Work out the finished part from the listing and answer in its coordinate system (mm). A direction names the side the tool comes from. Coordinates: 2 decimals unless noted, no trailing zeros. Write each loop counter-clockwise with the first axis right and the second up, starting at its lowest first coordinate (ties: lowest second). Pieces come first, ordered by that corner, then holes. Notation, with made-up numbers: (76, -8) - (80, -8) arc R23 cw to (80, 10) - close; hole circle Ø11 at (-29, 11.25). An arc over 180 degrees is marked (long way). Use a Markdown table: item, result. Add a question column.
(1) For a pull along X with two mould halves and no side action, classify faces 1 (the face through (25, -3, 0)), 2 (the face through (-3.923, -5.131, 0.113)), 3 (the face through (50, 0, 0)) as released by +X, released by -X, zero draft, split by the parting line, or undercut.
(2) The part is cut by section A-A, the plane x = 24. Give the vertices of the cut face in (y, z), then the cut area to 3 significant figures.
(3) A tool of negligible diameter and unlimited length cuts with its end or side. For faces 4 (the face through (0, 0.1, -3.4)), 5 (the face through (-1.972, 4.31, -2.535)), from which of +Z, -Z, +X, -X, +Y, -Y can it reach the whole face along a straight path? Write none if from no direction.
(4) Find the intervals of material crossed by line 1 (X direction, y = 3.25, z = 0.75); line 2 (Z direction, x = 21.5, y = 0); line 3 (X direction, y = -3, z = -0.75), in increasing order. Write a range as from..to.
(5) Given pin 1 Ø1.5 at (x, z) = (31.5, -2.5) entering from -Y; pin 2 Ø1.5 at (x, y) = (30, 1.5) entering from +Z; pin 3 Ø5 at (x, y) = (3, -4) entering from -Z, each flat-ended and moving along its own axis, determine where each tip first touches the part or whether it passes through.
Autodesk Inventor part; units mm, degrees
ref_plane "Work Plane1" through (1.525, 0, 0) normal (0, 0, 1) x (1, 0, 0)
ref_plane "YZ Plane" through (0, 0, 0) normal (1, 0, 0) x (0, 1, 0)
ref_plane "XZ Plane" through (0, 0, 0) normal (0, 1, 0) x (-1, 0, 0)
sketch "Sketch1" plane through (0, 0, 0) normal (0, 0, 1) x (1, 0, 0)
  line L0 (0, 3) -> (50, 3)
  line L1 (50, 3) -> (50, 0)
  line L2 (50, 0) -> (0, 0)
  line L3 (-10, 0) -> (60, 0)
  line L4 (0, -0.6) -> (0, 3.6)
  line L5 (0, 3) -> (0, 0)
  dimension "d2" = 6
  dimension "d59" = 50
revolve "Body" add sketch "Sketch1" angle 360 about axis through (50, 0, 0) along (-1, 0, 0)
sketch "Sketch2" plane through (0, 0, 0) normal (-1, 0, 0) x (0, 0, 1)
  line L0 (0, 5.7735) -> (5, 2.8868)
  line L1 (5, 2.8868) -> (5, -2.8868)
  line L2 (5, -2.8868) -> (0, -5.7735)
  line L3 (0, -5.7735) -> (-5, -2.8868)
  line L4 (-5, -2.8868) -> (-5, 2.8868)
  line L5 (-5, 2.8868) -> (0, 5.7735)
  line L6 (-7, 0) -> (7, 0)
  line L7 (0, 8.0829) -> (0, -8.0829)
  point P0 (0, 0)
  point P1 (0, 0)
  dimension "d11" = 10
extrude "Head" add sketch "Sketch2" along normal blind 4
sketch "Sketch4" plane through (0, 0, 0) normal (0, 0, 1) x (1, 0, 0)
  line L0 (-3.4226, 6) -> (-4, 5)
  line L1 (-1.1, 0) -> (-0.234, 0)
  line L2 (-4.7532, 0) -> (0.5192, 0)
  line L3 (-4, 6) -> (-3.4226, 6)
  line L4 (-4, 5) -> (-4, 6)
  line L5 (0, 7.2) -> (0, -1.2)
  dimension "d65" = 10
  dimension "d67" = 30
  dimension "d68" = 12
  dimension "d69" = 4
revolve "Chamfer1" cut sketch "Sketch4" angle 360 about axis through (-1.1, 0, 0) along (1, 0, 0)
thread "Thread"
chamfer "Chamfer2" distance 0.6135 distance2 0.6136 1 edges at (50, -3, 0) measured on face at (50, 0.3546, -0.935)
fillet "Fillet2" radius 0.25 1 edges at (0, -3, 0)
ref_plane "Work Plane1" through (1.525, 0, 0) normal (0, 0, 1) x (1, 0, 0)
equation "\"d2\" = GD"
equation "\"d59\" = NLG"
equation "\"d11\" = SW"
equation "\"d3\" = KOH"
equation "\"d71\" = RR"
equation "\"d15\" = GEL"
equation "\"d6\" = -0.5 * SPD + 0.5 * GD"
equation "\"d65\" = SW"
equation "\"d67\" = ANG1"
equation "\"d68\" = 1.2 * SW"
equation "\"d69\" = KOH"
equation "\"NLG\" = 50"
equation "\"GD\" = NND"
equation "\"BDM\" = NND"
equation "\"KOH\" = 4"
equation "\"GEL\" = 49"
equation "\"SW\" = 10"
equation "\"SPD\" = NND - 1.2269 * PTC"
equation "\"SD2\" = NND"
equation "\"SD\" = 0"
equation "\"ANG1\" = 30deg"
equation "\"GAL\" = 0.61345 * PTC"
equation "\"GUL\" = 0.61345 * PTC"
equation "\"RR\" = 0.25"
equation "\"RR1\" = 0.1"
equation "\"WFT\" = 0"
equation "\"GD1\" = THREADDIA - 1.2269 * PTC"
equation "\"THREADDIA\" = 6"
equation "\"TOA\" = 30deg"
equation "\"FAWI\" = 90deg"
equation "\"PTC\" = 1"
equation "\"NND\" = 6"
equation "\"E0\" = 1.155 * SW"
properties part number "Hexagon bolt GB/T 5781 M6 x 50" material "Steel, Mild"
Model answer:
| question | item | result |
|---|---|---|
| 1 | face 1 | zero draft |
| 1 | face 2 | released by -X |
| 1 | face 3 | released by +X |
| 2 | outline | circle Ø6 at (0, 0) |
| 2 | area | 28.3 mm^2 |
| 3 | face 4 | +X |
| 3 | face 5 | -Z, +X, -X, +Y |
| 4 | line 1 | -4..0 |
| 4 | line 2 | -3..3 |
| 4 | line 3 | -4..0.06 |
| 5 | pin 1 | y = -2.44 |
| 5 | pin 2 | z = 2.9 |
| 5 | pin 3 | z = -2.6 |
